from build123d import *

# Parameters (mm, degrees)
F1_DEPTH = 2.8


with BuildPart() as f1:
    # F0 (on Right) → F1 (new body)
    with BuildSketch(Plane.YZ):
        with BuildLine():
            Line((-26.111206, 5.284752), (-26.191802, 0))
            Line((-26.191802, 0), (-21.517237, 0))
            Line((-21.517237, 0), (-21.517237, 5.284752))
            Line((-21.517237, 5.284752), (-4.5604, 5.284752))
            Line((-4.5604, 5.284752), (-4.5604, 0))
            Line((-4.5604, 0), (-0.191802, 0))
            Line((-0.191802, 0), (-0.191802, 4.923995))
            ThreePointArc((-0.191802, 4.923995), (-0.132906, 5.235764), (0.180573, 5.284752))
            Line((0.180573, 5.284752), (3.02158, 5.284752))
            ThreePointArc((3.02158, 5.284752), (3.386548, 5.364985), (3.306315, 5.729954))
            Line((3.306315, 5.729954), (3.306315, 8.671706))
            ThreePointArc((3.306315, 8.671706), (3.3285, 9.0314), (3.686496, 9.072762))
            Line((3.686496, 9.072762), (9.408809, 9.072762))
            ThreePointArc((9.408809, 9.072762), (9.699169, 9.109567), (9.753991, 9.39707))
            Line((9.753991, 9.39707), (9.753991, 10.948542))
            ThreePointArc((9.753991, 10.948542), (9.792001, 11.210841), (9.529702, 11.248852))
            Line((9.529702, 11.248852), (2.258568, 11.248852))
            Line((2.258568, 11.248852), (1.22832, 11.248852))
            ThreePointArc((1.22832, 11.248852), (0.908223, 11.188042), (0.969033, 10.867945))
            Line((0.969033, 10.867945), (0.969033, 9.437368))
            ThreePointArc((0.969033, 9.437368), (0.978366, 9.136595), (0.684297, 9.072762))
            Line((0.684297, 9.072762), (-26.857296, 9.072762))
            ThreePointArc((-26.857296, 9.072762), (-26.867436, 9.072625), (-26.877575, 9.072762))
            ThreePointArc((-26.877575, 9.072762), (-27.118402, 9.168825), (-27.239549, 9.398061))
            ThreePointArc((-27.239549, 9.398061), (-27.242897, 9.448086), (-27.239549, 9.498111))
            Line((-27.239549, 9.498111), (-27.239549, 10.646189))
            ThreePointArc((-27.239549, 10.646189), (-27.404115, 11.017522), (-27.737966, 11.248852))
            Line((-27.737966, 11.248852), (-28.227659, 11.248852))
            Line((-28.227659, 11.248852), (-35.302914, 11.248852))
            ThreePointArc((-35.302914, 11.248852), (-35.522633, 11.267151), (-35.540933, 11.047432))
            Line((-35.540933, 11.047432), (-35.540933, 9.410823))
            Line((-35.540933, 9.410823), (-35.540933, 9.282929))
            ThreePointArc((-35.540933, 9.282929), (-35.455206, 9.140153), (-35.302914, 9.072762))
            Line((-35.302914, 9.072762), (-31.523069, 9.072762))
            ThreePointArc((-31.523069, 9.072762), (-31.44012, 9.083231), (-31.357172, 9.072762))
            ThreePointArc((-31.357172, 9.072762), (-31.187614, 8.967777), (-31.108157, 8.784861))
            ThreePointArc((-31.108157, 8.784861), (-31.106266, 8.749376), (-31.108157, 8.713891))
            Line((-31.108157, 8.713891), (-31.108157, 5.670374))
            Line((-31.108157, 5.670374), (-31.108157, 5.63826))
            ThreePointArc((-31.108157, 5.63826), (-30.999114, 5.391756), (-30.75172, 5.284752))
            Line((-30.75172, 5.284752), (-26.111206, 5.284752))
        make_face()
        with BuildLine():
            ThreePointArc((-31.108157, 5.670374), (-31.108506, 5.654317), (-31.108157, 5.63826))
            Line((-31.108157, 5.63826), (-31.108157, 5.670374))
        make_face()
        with BuildLine():
            Line((-31.108157, 8.784861), (-31.108157, 8.713891))
            ThreePointArc((-31.108157, 8.713891), (-31.106266, 8.749376), (-31.108157, 8.784861))
        make_face()
        with BuildLine():
            Line((-31.523069, 9.072762), (-31.357172, 9.072762))
            ThreePointArc((-31.357172, 9.072762), (-31.44012, 9.083231), (-31.523069, 9.072762))
        make_face()
        with BuildLine():
            ThreePointArc((-35.540933, 9.410823), (-35.548449, 9.346876), (-35.540933, 9.282929))
            Line((-35.540933, 9.282929), (-35.540933, 9.410823))
        make_face()
        with BuildLine():
            ThreePointArc((-27.737966, 11.248852), (-27.982812, 11.289888), (-28.227659, 11.248852))
            Line((-28.227659, 11.248852), (-27.737966, 11.248852))
        make_face()
        with BuildLine():
            Line((-27.239549, 9.398061), (-27.239549, 9.498111))
            ThreePointArc((-27.239549, 9.498111), (-27.242897, 9.448086), (-27.239549, 9.398061))
        make_face()
        with BuildLine():
            Line((-26.857296, 9.072762), (-26.877575, 9.072762))
            ThreePointArc((-26.877575, 9.072762), (-26.867436, 9.072625), (-26.857296, 9.072762))
        make_face()
    extrude(amount=F1_DEPTH)


solid = f1.part
Check sheet for the modelled part. Datum: model origin and axes. Units: mm. A direction names the side the tool comes from. Give positions to 0.01 mm unless a question says otherwise; leave off trailing zeros. Write each loop counter-clockwise with the first axis right and the second up, starting at its lowest first coordinate (ties: lowest second). Pieces come first, ordered by that corner, then holes. Notation, with made-up numbers: M 7.25,28.5 L 44.25,28.5 A29 cw 44.25,55.5 Z; hole C 81,5.25 d4. An arc over 180 degrees is marked long. Use one line per item in the form item = value.
(1) Section check C-C on z = 6.25. Record the boundary of the cut face in (x, y), plus the area to 3 significant figures.
Answer block:
outline = M 0,-31.11 L 2.8,-31.11 L 2.8,3.31 L 0,3.31 Z
area = 96.4 mm2
(2) Depth check by flat-ended pin: P1, Ø1.4, axis at x = 2, y = -14, coming from the +Z side; P2, Ø1.4, axis at x = 1, y = -31, coming from the +Z side; P3, Ø0.8, axis at x = 1, z = 10.5, coming from the -Y side. Enter the tip coordinate at first touch or a pass-through.
Answer block:
P1 = 9.07
P2 = 11.25
P3 = -35.54
(3) Tool access check on faces 1 (the flat face through (1, 7, 9.073)), 2 (the flat face through (1, 0.969, 10)), 3 (the flat face through (1, -0.192, 2)), 4 (the flat face through (1, -32, 11.249)), 5 (the flat face through (1, -33, 9.073)). Record the directions out of +Z, -Z, +X, -X, +Y, -Y that give a thin tool (end or side, any length) a straight path to the whole face; none if there is none.
Answer block:
face_1 = -Z, +X, -X
face_2 = +X, -X
face_3 = -Z, +X, -X, +Y
face_4 = +Z, +X, -X
face_5 = -Z, +X, -X, -Y
(4) Section check A-A on z = 3. Record the boundary of the cut face in (x, y), plus the area to 3 significant figures.
Answer block:
outline = M 0,-26.15 L 2.8,-26.15 L 2.8,-21.52 L 0,-21.52 Z; M 0,-4.56 L 2.8,-4.56 L 2.8,-0.19 L 0,-0.19 Z
area = 25.2 mm2
(5) Section check B-B on y = -23. Record the boundary of the cut face in (x, z).
Answer block:
outline = M 0,0 L 2.8,0 L 2.8,9.07 L 0,9.07 Z
(6) Material ranges on line 1 along Y through (x, z) = (1.5, 10.5); line 2 along Y through (x, z) = (2.45, 0.5); line 3 along Z through (x, y) = (1.35, -23), recorded low to high.
Answer block:
line_1 = -35.54 to -27.24, 0.97 to 9.75
line_2 = -26.18 to -21.52, -4.56 to -0.19
line_3 = 0 to 9.07
(7) Draft check along Y on faces 6 (the flat face through (1, 2, 5.285)), 7 (the flat face through (1, 3.306, 7)), 8 (the flat face through (1, -21.517, 3)), 9 (the flat face through (1, -24, 0)). Enter one of: pulls with the +Y half, pulls with the -Y half, needs draft (parallel to the pull), parting line crosses it, or undercut.
Answer block:
face_6 = undercut
face_7 = pulls with the +Y half
face_8 = undercut
face_9 = needs draft
